Can you work these out from the model? Positions are in its coordinate system, mm. Face numbers are marked on the shaded views. A direction names the side the tool comes from. Give positions to 0.01 mm unless a question says otherwise; leave off trailing zeros. Order: outer loops, then holes, each group sorted by start corner. A loop starts at its lowest first (then second) coordinate and runs counter-clockwise, first axis right, second up. Notation, with made-up numbers: (64, 88) - (93, 88) arc R19 cw to (93, 104) - close; hole circle Ø5 at (19.25, 52). An arc over 180 degrees is marked (long way). Answer as a JSON object with one key per item and string values.
```python
from build123d import *

# Parameters (mm, degrees)
SKETCH1_R                = 8
SKETCH1_R_2              = 3.5
BOSS_EXTRUDE1_DEPTH      = 3
SKETCH2_R                = 8
SKETCH2_R_2              = 5
BOSS_EXTRUDE2_DEPTH      = 6
WRAP3_SECTION_W          = 4
WRAP3_SECTION_H          = 2
WRAP3_ANGLE              = 57.295779513
WRAP3_SECTOR_2_SECTION_W = 4
WRAP3_SECTOR_2_SECTION_H = 2
WRAP3_SECTOR_2_ANGLE     = 57.295779513
CUT_EXTRUDE1_DEPTH       = 4
BOSS_EXTRUDE3_DEPTH      = 9


with BuildPart() as part:
    # Sketch1 → Boss-Extrude1 (new body)
    with BuildSketch(Plane.XY):
        Circle(SKETCH1_R)
        Circle(SKETCH1_R_2, mode=Mode.SUBTRACT)
    extrude(amount=BOSS_EXTRUDE1_DEPTH)

    # Sketch2 → Boss-Extrude2 (add)
    with BuildSketch(Plane.XY.offset(3)):
        Circle(SKETCH2_R)
        Circle(SKETCH2_R_2, mode=Mode.SUBTRACT)
    extrude(amount=BOSS_EXTRUDE2_DEPTH)

    # Wrap3 section (on wrap section) → Wrap3 (revolve, cut)
    with BuildSketch(Plane(origin=(0, 0, 0), x_dir=(-0.8779640629990781, -0.4787265441587198, 0), z_dir=(0.4787265441587198, -0.8779640629990781, 0))):
        with Locations((6, -8)):
            Rectangle(WRAP3_SECTION_W, WRAP3_SECTION_H)
    revolve(axis=Axis((0, 0, 0), (0, 0, -1)), revolution_arc=WRAP3_ANGLE, mode=Mode.SUBTRACT)

    # Wrap3 sector 2 section (on wrap section) → Wrap3 sector 2 (revolve, cut)
    with BuildSketch(Plane(origin=(0, 0, 0), x_dir=(0.8772005042746819, 0.4801242290285337, 0), z_dir=(-0.4801242290285337, 0.8772005042746819, 0))):
        with Locations((6, -8)):
            Rectangle(WRAP3_SECTOR_2_SECTION_W, WRAP3_SECTOR_2_SECTION_H)
    revolve(axis=Axis((0, 0, 0), (0, 0, -1)), revolution_arc=WRAP3_SECTOR_2_ANGLE, mode=Mode.SUBTRACT)

    # Sketch5 → Cut-Extrude1 (cut)
    with BuildSketch(Plane(origin=(0, 0, 0), x_dir=(-1, 0, 0), z_dir=(0, 0, -1))):
        with BuildLine():
            Line((-1.5, 6.837397166), (-1.5, 7.858116823))
            ThreePointArc((-1.5, 7.858116823), (0, -8), (1.5, 7.858116823))
            Line((1.5, 7.858116823), (1.5, 6.837397166))
            ThreePointArc((1.5, 6.837397166), (0, -7), (-1.5, 6.837397166))
        make_face()
    extrude(amount=-CUT_EXTRUDE1_DEPTH, mode=Mode.SUBTRACT)

    # Sketch6 → Boss-Extrude3 (add)
    with BuildSketch(Plane(origin=(0, 0, 0), x_dir=(-1, 0, 0), z_dir=(0, 0, -1))):
        with BuildLine():
            Line((-1.5, 7.858116823), (-1.5, 8.837397166))
            Line((-1.5, 8.837397166), (1.5, 8.837397166))
            Line((1.5, 8.837397166), (1.5, 7.858116823))
            ThreePointArc((1.5, 7.858116823), (0, 8), (-1.5, 7.858116823))
        make_face()
    extrude(amount=-BOSS_EXTRUDE3_DEPTH)


solid = part.part
```
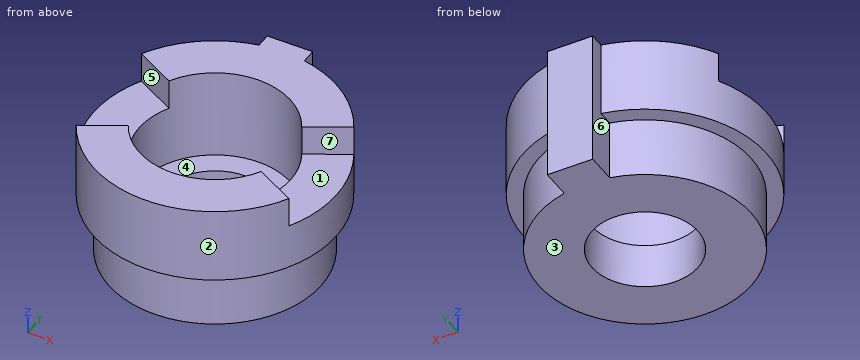
Q1. If we section it at B-B, the plane y = 0: Please give me the cut outline in (x, z), then the cut area to 3 significant figures.
Recorded:
{"outline": "(-8, 4) - (-7, 4) - (-7, 0) - (-3.5, 0) - (-3.5, 3) - (-5, 3) - (-5, 7) - (-8, 7) - close; (3.5, 0) - (7, 0) - (7, 4) - (8, 4) - (8, 7) - (5, 7) - (5, 3) - (3.5, 3) - close", "area": "43.0 mm^2"}
Q2. If we section it at D-D, the plane z = 3.5: Please give me the cut outline in (x, y).
Recorded:
{"outline": "(-1.5, 6.84) arc R7 ccw (long way) to (1.5, 6.84) - (1.5, 8.84) - (-1.5, 8.84) - close; hole circle Ø10 at (0, 0)"}
Q3. If we section it at A-A, the plane z = 8: Please give me the cut outline in (x, y).
Recorded:
{"outline": "(-7.02, -3.83) arc R8 ccw to (7.02, -3.83) - (4.39, -2.39) arc R5 cw to (-4.39, -2.39) - close; (-7.02, 3.84) - (-4.39, 2.4) arc R5 cw to (4.39, 2.4) - (7.02, 3.84) arc R8 ccw to (1.5, 7.86) - (1.5, 8.84) - (-1.5, 8.84) - (-1.5, 7.86) arc R8 ccw to start"}
Q4. If we section it at C-C, the plane x = 0: Please give me the cut outline in (y, z).
Recorded:
{"outline": "(-8, 4) - (-7, 4) - (-7, 0) - (-3.5, 0) - (-3.5, 3) - (-5, 3) - (-5, 9) - (-8, 9) - close; (3.5, 0) - (8.84, 0) - (8.84, 9) - (5, 9) - (5, 3) - (3.5, 3) - close"}
Q5. We'd pull the mould along Y, two halves only. Please class the marked faces 1, 2 and 3: released by +Y, released by -Y, zero draft, split by the parting line, or undercut.
Recorded:
{"face 1": "undercut", "face 2": "split by the parting line", "face 3": "zero draft"}
Q6. I'm going to push flat-ended pins straight in: pin 1 Ø3 at (x, y) = (6.5, -1) entering from +Z; pin 2 Ø2 at (y, z) = (3, 6.5) entering from +X; pin 3 Ø5.5 at (x, y) = (0, 0) entering from +Z; pin 4 Ø0.6 at (y, z) = (8, 2.5) entering from -X. Where does each tip first touch, or does it pass through?
Recorded:
{"pin 1": "stops at z = 7", "pin 2": "stops at x = 7.75", "pin 3": "passes through", "pin 4": "stops at x = -1.5"}
Q7. Which directions (+Z, -Z, +X, -X, +Y, -Y) give clear straight access to the entire face, cutting with the end or side of a thin tool? Please do the marked faces 4, 5, 6 and 7.
Recorded:
{"face 4": "+Z", "face 5": "+Z, -X", "face 6": "-Z, -X, +Y", "face 7": "+Z, +X"}
Q8. I need wall thicknesses on L1, parallel to Y at x = 0, z = 2; L2, parallel to Y at x = 0, z = 4.35; L3, parallel to X at y = 0, z = 6.3. Which ranges of each line are inside material? Lowest first, please.
Recorded:
{"L1": "y = -7 to -3.5, 3.5 to 8.84", "L2": "y = -8 to -5, 5 to 8.84", "L3": "x = -8 to -5, 5 to 8"}
